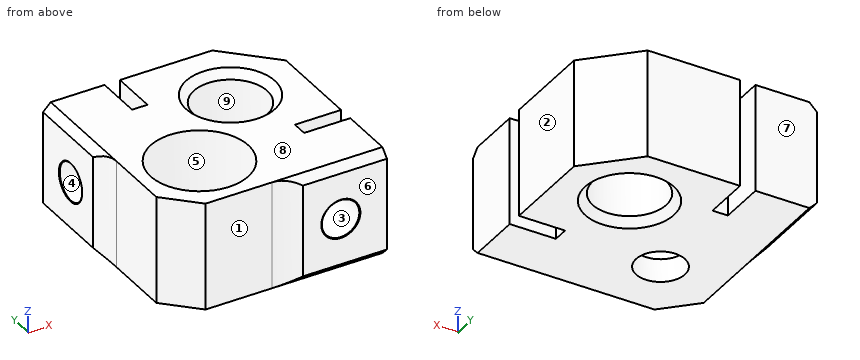
Autodesk Inventor part; units mm, degrees
ref_plane "YZ Plane" through (0, 0, 0) normal (1, 0, 0) x (0, 1, 0)
ref_plane "XZ Plane" through (0, 0, 0) normal (0, 1, 0) x (-1, 0, 0)
ref_plane "XY Plane" through (0, 0, 0) normal (0, 0, 1) x (1, 0, 0)
sketch "Sketch1" plane through (0, 0, 0) normal (0, 0, 1) x (1, 0, 0)
  line L0 (0, 0) -> (14, 0)
  line L1 (14, 0) -> (14, 14)
  line L2 (14, 14) -> (0, 14)
  line L3 (0, 14) -> (0, 0)
  dimension "d0" = 14
  dimension "d1" = 14
extrude "Extrusion1" add sketch "Sketch1" along normal mid plane 7
hole "Hole1" at (9.5, 9.5, 3.5) direction (0, 0, -1) diameter 4.7752 end through all
sketch "Sketch22" plane through (0, 0, 3.5) normal (0, 0, 1) x (1, 0, 0)
  line L0 (0, 0) -> (0, 14)
  line L1 (14, 0) -> (0, 0)
  arc A0 (0.5, 0) -> (0, 0.5) centre (0, 0) ccw
  line L2 (0, 0.5) -> (0, 0)
  line L3 (0, 0) -> (0.5, 0)
  dimension "d145" = 0.5
extrude "Extrusion19" cut sketch "Sketch22" against normal through all
sketch "Sketch15" plane through (0, 0, 3.5) normal (0, 0, 1) x (1, 0, 0)
  line L0 (14, 0) -> (0, 0)
  line L1 (0, 0) -> (0, 14)
  line L2 (5, 5) -> (5, 12)
  line L3 (5, 12) -> (4, 12)
  line L4 (4, 12) -> (4, 5)
  line L5 (5, 4) -> (12, 4)
  line L6 (12, 4) -> (12, 5)
  line L7 (12, 5) -> (5, 5)
  arc A0 (0.5, 0) -> (0, 0.5) centre (0, 0) ccw
  line L8 (4, 5) -> (0, 5)
  line L9 (0, 5) -> (0, 0)
  line L10 (0, 0) -> (5, 0)
  line L11 (5, 0) -> (5, 4)
  point P0 (0, 7.5)
  point P1 (7.5, 0)
  point P2 (0.315, 0.3883)
  dimension "d94" = 1
  dimension "d95" = 4
  dimension "d96" = 4
  dimension "d97" = 12
extrude "sawblade" [suppressed]
chamfer "Chamfer5" distance 3 angle 45 1 edges at (14, 14, 0)
chamfer "Chamfer8" distance 0.5 angle 45 4 edges at (7.25, 0, 3.5) (0, 7.25, 3.5) (7.25, 0, -3.5) (0, 7.25, -3.5)
chamfer "Chamfer9" distance 0.5 angle 45 2 edges at (9.5, 11.8876, 3.5) (9.5, 11.8876, -3.5)
hole "Hole6" at (11, 0, 0) direction (0, 1, 0) diameter 2.4384 depth 8 tip angle 118 countersink diameter 2.54 countersink angle 120
hole "Hole7" at (0, 11, 0) direction (1, 0, 0) diameter 2.4384 depth 8 tip angle 118 countersink diameter 2.54 countersink angle 120
sketch "Sketch25" plane through (0, 0, 3.5) normal (0, 0, 1) x (1, 0, 0)
  line L0 (0.5, 14) -> (11, 14)
  line L1 (5, 14) -> (4, 14)
  line L2 (4, 14) -> (4, 11)
  line L3 (4, 11) -> (5, 11)
  line L4 (5, 11) -> (5, 14)
  line L5 (0, 14) -> (0, 0.5)
  point P0 (0, 0)
  dimension "d183" = 3
  dimension "d184" = 4
  dimension "d185" = 1
extrude "sawblade1" cut sketch "Sketch25" against normal through all
sketch "Sketch26" plane through (0, 0, 3.5) normal (0, 0, 1) x (1, 0, 0)
  line L0 (14, 5) -> (11, 5)
  line L1 (11, 5) -> (11, 4)
  line L2 (11, 4) -> (14, 4)
  line L3 (14, 4) -> (14, 5)
  line L4 (0.5, 0) -> (14, 0)
  point P0 (0, 0)
  dimension "d188" = 4
  dimension "d189" = 1
  dimension "d190" = 3
extrude "sawblade2" cut sketch "Sketch26" against normal through all
hole "Hole8" [suppressed]
hole "Hole9" [suppressed]
hole "Hole10" at (4.5, 4.5, 3.5) direction (0, 0, -1) diameter 6.35 depth 5.5
sketch "Sketch27" plane through (0, 0, 3.5) normal (0, 0, 1) x (1, 0, 0)
  line L0 (2.5, 0.5) -> (6.825, 0.5)
  line L1 (10, -2.675) -> (10, -7.675)
  line L2 (10, -7.675) -> (-7.675, -7.675)
  line L3 (-7.675, -7.675) -> (-7.675, 10)
  line L4 (-7.675, 10) -> (-2.675, 10)
  arc A0 (10, -2.675) -> (6.825, 0.5) centre (6.825, -2.675) ccw
  arc A1 (0.5, 6.825) -> (-2.675, 10) centre (-2.675, 6.825) ccw
  line L5 (0.5, 2.5) -> (0.5, 6.825)
  line L6 (2.5, 0.5) -> (0.5, 2.5)
  point P0 (0, 0)
  point P1 (0.5, 0.5)
  dimension "d220" = 3.175
  dimension "d222" = 0.5
  dimension "d223" = 0.5
  dimension "d225" = 5
  dimension "d226" = 2
  dimension "d227" = 2
  dimension "d228" = 10
extrude "Extrusion24" cut sketch "Sketch27" against normal through all
hole "Hole11" at (4.5, 4.5, -2) direction (0, 0, -1) diameter 3.175 end through all
properties part number "FOX-ME-118-03" material "Delrin, Black"
Could you check a few things on this model? Use its own coordinates, in mm. Face numbers are marked on the shaded views. A direction names the side the tool comes from. Give positions to 0.01 mm unless a question says otherwise; leave off trailing zeros. Order: outer loops, then holes, each group sorted by start corner. A loop starts at its lowest first (then second) coordinate and runs counter-clockwise, first axis right, second up. Notation, with made-up numbers: M 63.25,-36.75 L 103.25,-36.75 A18 cw 103.25,-17.75 Z; hole C -5.5,52 d6. An arc over 180 degrees is marked long. One line per question, with ' | ' between items.
1. We'd pull the mould along Y, two halves only. Please class the marked faces 6, 7, 8 and 9: +Y half, -Y half, draft (parallel to the pull), parting line (faces both ways), or undercut.
Results:
face 6: -Y half | face 7: +Y half | face 8: draft | face 9: undercut
2. I want a section at D-D (z = 2.5). List the corners of the cut face in (x, y) for me (3 decimals), and give its area (3 significant figures).
Results:
outline: M 0,8.535 A3.175 cw 0.5,6.825 L 0.5,2.5 L 2.5,0.5 L 6.825,0.5 A3.175 cw 8.535,0 L 14,0 L 14,4 L 11,4 L 11,5 L 14,5 L 14,11 L 11,14 L 5,14 L 5,11 L 4,11 L 4,14 L 0,14 Z; hole C 4.5,4.5 d6.35; hole C 9.5,9.5 d4.775 | area: 126 mm²
3. For the marked faces 1, 2, 3, 4 and 5, which set-ups out of +Z, -Z, +X, -X, +Y, -Y let a thin tool reach every point of the face, with its end or its side?
Results:
face 1: +Z, -Z, -X, -Y | face 2: +Z, -Z, +X, +Y, -Y | face 3: -Y | face 4: -X | face 5: +Z
4. I'm going to push flat-ended pins straight in: pin 1 (0.8 mm diameter, centred on x = 4.5, z = 2, fed in from +Y); pin 2 (2 mm diameter, centred on y = 5, z = 1.5, fed in from -X); pin 3 (0.8 mm diameter, centred on y = 4.5, z = -2.5, fed in from +X). Where does each tip first touch, or does it pass through?
Results:
pin 1: y = 11 | pin 2: x = 0.5 | pin 3: x = 11
5. I want a section at A-A (x = 13.25). List the corners of the cut face in (y, z) for me, and give its area (3 significant figures).
Results:
outline: M 0,-3 L 0.5,-3.5 L 4,-3.5 L 4,3.5 L 0.5,3.5 L 0,3 Z; M 5,-3.5 L 11.75,-3.5 L 11.75,3.5 L 5,3.5 Z | area: 75.0 mm²
6. If I drill on line 1 (Y direction, x = 4.5, z = -3); line 2 (X direction, y = 9.5, z = -1.25); line 3 (Z direction, x = 2.25, y = 11), over which ranges is the centre line in solid material (lowest first)?
Results:
line 1: 0.5 to 2.91, 6.09 to 11 | line 2: 0 to 7.11, 11.89 to 14 | line 3: -3.5 to -1.22, 1.22 to 3.5
7. I want a section at B-B (z = 0). Give the number of separate pieces and of enclosed holes in the cut face, and give its area (3 significant figures).
Results:
separate pieces: 4 | enclosed holes: 1 | area: 91.1 mm²
8. I want a section at C-C (y = 5.75). List the corners of the cut face in (x, z) for me.
Results:
outline: M 0.5,-3.5 L 3.52,-3.5 L 3.52,-2 L 1.58,-2 L 1.58,3.5 L 0.5,3.5 Z; M 5.48,-3.5 L 14,-3.5 L 14,3.5 L 7.42,3.5 L 7.42,-2 L 5.48,-2 Z; hole C 11,0 d2.44
